Work out the finished part from the listing and answer in its coordinate system (mm). A direction names the side the tool comes from. Give positions to 0.01 mm unless a question says otherwise; leave off trailing zeros. Order: outer loops, then holes, each group sorted by start corner. A loop starts at its lowest first (then second) coordinate and runs counter-clockwise, first axis right, second up.
Autodesk Inventor part; units mm, degrees
ref_plane "YZ Plane" through (0, 0, 0) normal (1, 0, 0) x (0, 1, 0)
ref_plane "XZ Plane" through (0, 0, 0) normal (0, 1, 0) x (-1, 0, 0)
ref_plane "XY Plane" through (0, 0, 0) normal (0, 0, 1) x (1, 0, 0)
sketch "Sketch1" plane through (0, 0, 0) normal (0, 0, 1) x (1, 0, 0)
  line L0 (0, 0) -> (0, 4)
  line L1 (0, 4) -> (0.36, 4)
  line L2 (0.36, 4) -> (2.36, 2)
  line L3 (2.36, 2) -> (10, 2)
  line L4 (10, 2) -> (10, 0)
  line L5 (10, 0) -> (0, 0)
  dimension "d0" = 4
  dimension "d1" = 0.36
  dimension "d2" = 135
  dimension "d3" = 10
  dimension "d4" = 2
revolve "Revolution1" add sketch "Sketch1" angle 360 about axis through (10, 0, 0) along (-1, 0, 0)
chamfer "Chamfer1" distance 0.5 angle 45 1 edges at (10, -2, 0)
sketch "Sketch2" plane through (0, 0, 0) normal (-1, 0, 0) x (0, 0, 1)
  circle A0 centre (0, 0) radius 4
  line L0 (-1.4434, 0) -> (-0.7217, 1.25)
  line L1 (-0.7217, 1.25) -> (0.7217, 1.25)
  line L2 (0.7217, 1.25) -> (1.4434, 0)
  line L3 (1.4434, 0) -> (0.7217, -1.25)
  line L4 (0.7217, -1.25) -> (-0.7217, -1.25)
  line L5 (-0.7217, -1.25) -> (-1.4434, 0)
  dimension "d9" = 2.5
extrude "Extrusion1" cut sketch "Sketch2" against normal blind 1.5 contours L0 L1 L2 L3 L4 L5
thread "Thread1"
properties part number "FHS4x10" material "Steel, Alloy"
1. The mould has two halves that part along Y. Classify faces 4 (the face through (0, 2, 0)), 5 (the face through (1.5, 0, 0)), 6 (the face through (0.74, 0.616, -1.088)), 7 (the face through (2.2, -0.5, 2.1)): pulls with the +Y half, pulls with the -Y half, needs draft (parallel to the pull), parting line crosses it, or undercut.
Findings below:
face 4: needs draft
face 5: undercut
face 6: undercut
face 7: parting line crosses it
2. The part is cut by section C-C (x = 5). Write down the section's boundary in (y, z).
Findings below:
outline: circle Ø4 at (0, 0)
3. Which of the six approach directions +Z, -Z, +X, -X, +Y, -Y give full straight-line access (tool end or side, diameter ignored) to faces 1 (the face through (0.183, -0.867, -3.905)), 2 (the face through (6, 0, -2)), 3 (the face through (0.74, -0.63, -1.08))?
Findings below:
face 1: +X, -X
face 2: +X
face 3: -X
4. Given P1, Ø3, axis at y = 3, z = 3, coming from the +X side; P2, Ø1.5, axis at x = 4, z = -1, coming from the -Y side, each flat-ended and moving along its own axis, determine where each tip first touches the part or whether it passes through.
Findings below:
P1: stops at x = 1.62
P2: stops at y = -1.98
5. The part is cut by section B-B (x = 2). Write down the section's boundary in (y, z), then the cut area to 3 significant figures.
Findings below:
outline: circle Ø4.72 at (0, 0)
area: 17.5 mm2
6. The part is cut by section A-A (z = 0). Write down the section's boundary in (x, y), then the cut area to 3 significant figures.
Findings below:
outline: (0, -4) - (0.36, -4) - (2.36, -2) - (9.5, -2) - (10, -1.5) - (10, 1.5) - (9.5, 2) - (2.36, 2) - (0.36, 4) - (0, 4) - (0, 1.25) - (1.5, 1.25) - (1.5, -1.25) - (0, -1.25) - close
area: 41.4 mm2
7. Straight lines are drawn through the part: probe 1 along X at (y, z) = (1.5, -2.5); probe 2 along Z at (x, y) = (1, 0.75); probe 3 along Z at (x, y) = (9.25, -0.5). For each, find the intervals that lie inside material, in ascending order.
Findings below:
probe 1: x = 0 to 1.44
probe 2: z = -3.28 to -1.01, 1.01 to 3.28
probe 3: z = -1.94 to 1.94
